Answer from the drawing. Dimensions are ordinates in mm from the lowest x, y and z of the part. A direction names the side the tool comes from. Give positions to 0.01 mm unless a question says otherwise; leave off trailing zeros. Write each loop counter-clockwise with the first axis right and the second up, starting at its lowest first coordinate (ties: lowest second). Pieces come first, ordered by that corner, then holes.
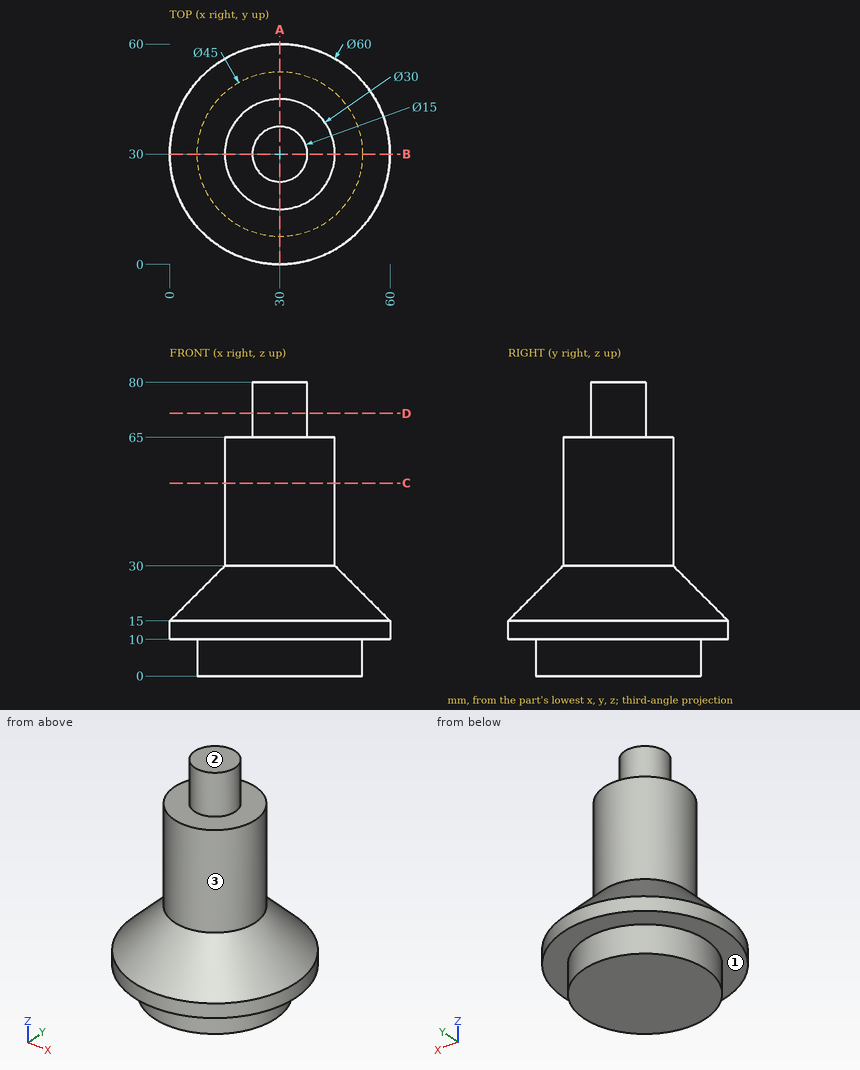
Item 1: Section C-C (z = 52.5) is taken. Write down the section's boundary in (x, y).
Result set:
outline: circle Ø30 at (30, 30)
Item 2: Find the intervals of material crossed by line 1 along Z through (x, y) = (42.5, 23); line 2 along X through (y, z) = (28, 68.5); line 3 along Y through (x, z) = (42, 7.5), in increasing order.
Result set:
line 1: z = 0 to 65
line 2: x = 22.77 to 37.23
line 3: y = 10.97 to 49.03
Item 3: Which of the six approach directions +Z, -Z, +X, -X, +Y, -Y give full straight-line access (tool end or side, diameter ignored) to the marked faces 1, 2 and 3?
Result set:
face 1: -Z
face 2: +Z, +X, -X, +Y, -Y
face 3: +Z
Item 4: Section D-D (z = 71.5) is taken. Write down the section's boundary in (x, y), and give its area (3 significant figures).
Result set:
outline: circle Ø15 at (30, 30)
area: 177 mm2
Item 5: Section A-A (x = 30) is taken. Write down the section's boundary in (y, z), and give its area (3 significant figures).
Result set:
outline: (0, 10) - (7.5, 10) - (7.5, 0) - (52.5, 0) - (52.5, 10) - (60, 10) - (60, 15) - (45, 30) - (45, 65) - (37.5, 65) - (37.5, 80) - (22.5, 80) - (22.5, 65) - (15, 65) - (15, 30) - (0, 15) - close
area: 2,700 mm2
Item 6: Each of these flat-tipped pins is pushed along its axis until it touches: pin 1 Ø2 at (x, z) = (22.5, 45) entering from +Y; pin 2 Ø6 at (y, z) = (39, 32.5) entering from -X; pin 3 Ø1.5 at (y, z) = (29.5, 45.5) entering from -X; pin 4 Ø18 at (x, y) = (44.5, 28.5) entering from -Z. Where does it stop, or does it pass through?
Result set:
pin 1: stops at y = 43.52
pin 2: stops at x = 16.25
pin 3: stops at x = 15
pin 4: stops at z = 0
